Study the drawing (mm; zero at the part's minimum x, y, z) and answer. Coordinates: 2 decimals unless noted, no trailing zeros. Loops run counter-clockwise (first coordinate to the right, second up) from the corner with the lowest first, then second, coordinate; pieces in that order, holes last. Notation, with made-up numbers: (75.5, -29.75) -> (122.5, -29.75) arc R22 ccw to (122.5, -21.75) -> close; hole circle Ø8 at (-19.75, 5). An arc over 180 degrees is marked (long way). Answer as CSV lines item,"result".
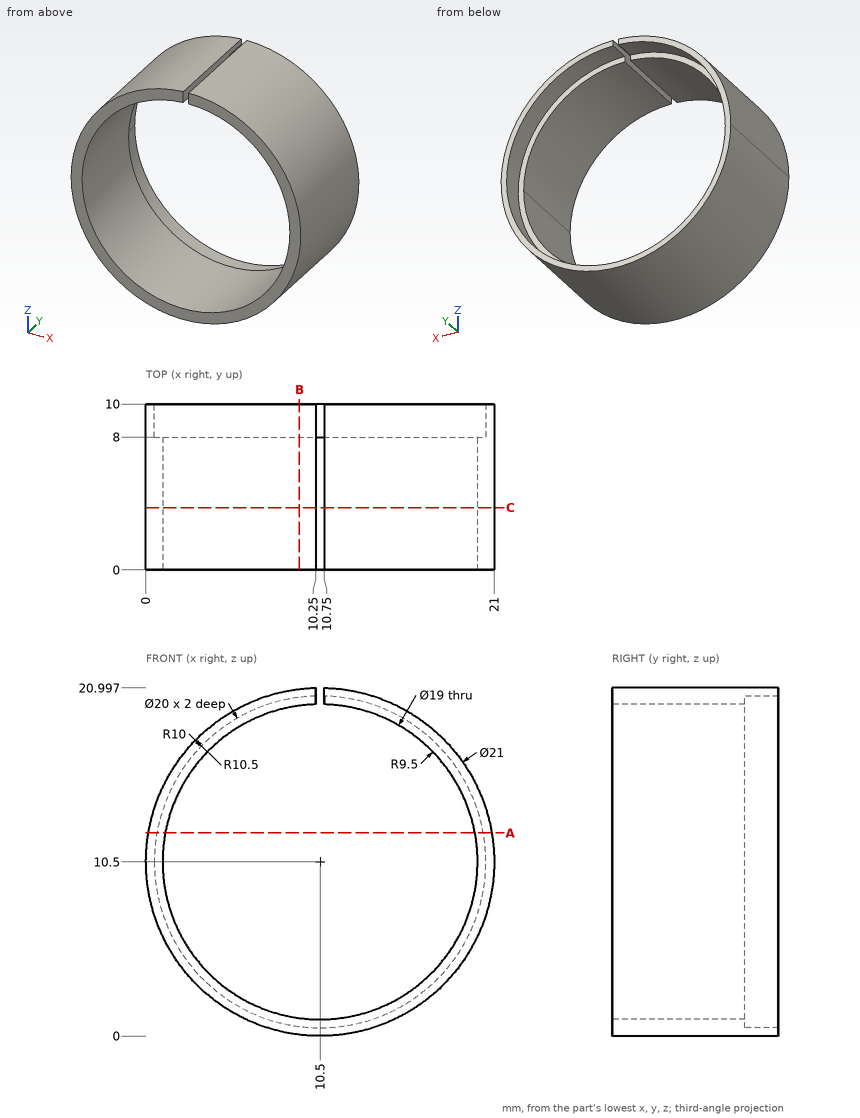
Q1. A cutting plane is placed at A-A, the plane z = 12.25. Write down the section's boundary in (x, y).
Results:
outline,"(0.15, 0) -> (1.16, 0) -> (1.16, 8) -> (0.65, 8) -> (0.65, 10) -> (0.15, 10) -> close; (19.84, 0) -> (20.85, 0) -> (20.85, 10) -> (20.35, 10) -> (20.35, 8) -> (19.84, 8) -> close"
Q2. Find the intervals of material crossed by probe 1 along X at (y, z) = (3, 10.5); probe 2 along X at (y, z) = (8.85, 10.5); probe 3 along Z at (x, y) = (7.75, 6.75), in increasing order. Write a range as [from, to].
Results:
probe 1,"x = [0, 1], [20, 21]"
probe 2,"x = [0, 0.5], [20.5, 21]"
probe 3,"z = [0.37, 1.41], [19.59, 20.63]"
Q3. Given pin 1 Ø1 at (x, y) = (6, 3.5) entering from +Z; pin 2 Ø6 at (x, y) = (8.5, 6.5) entering from +Z; pin 3 Ø5 at (x, y) = (18, 3.5) entering from -Z; pin 4 Ø4 at (x, y) = (6.5, 2.5) entering from +Z, each flat-ended and moving along its own axis, determine where each tip first touches the part or whether it passes through.
Results:
pin 1,"stops at z = 20.21"
pin 2,"stops at z = 21"
pin 3,"stops at z = 1.27"
pin 4,"stops at z = 20.81"
Q4. A cutting plane is placed at C-C, the plane y = 3.75. Write down the section's boundary in (x, z), and give its area (3 significant figures).
Results:
outline,"(10.25, 20) -> (10.25, 21) arc R10.5 ccw (long way) to (10.75, 21) -> (10.75, 20) arc R9.5 cw (long way) to start"
area,"62.3 mm²"
Q5. A cutting plane is placed at B-B, the plane x = 9.25. Write down the section's boundary in (y, z), and give its area (3 significant figures).
Results:
outline,"(0, 0.07) -> (10, 0.07) -> (10, 0.58) -> (8, 0.58) -> (8, 1.08) -> (0, 1.08) -> close; (0, 19.92) -> (8, 19.92) -> (8, 20.42) -> (10, 20.42) -> (10, 20.93) -> (0, 20.93) -> close"
area,"18.1 mm²"
